Design review of the part built by this model. Coordinates are the model's own, in mm. A direction names the side the tool comes from. Coordinates: 2 decimals unless noted, no trailing zeros. Order: outer loops, then holes, each group sorted by start corner. A loop starts at its lowest first (then second) coordinate and runs counter-clockwise, first axis right, second up. Notation, with made-up numbers: M 82.25,-19.75 L 113.25,-19.75 A24 ccw 113.25,-8.75 Z; hole C 62.25,-13 d4. An arc over 180 degrees is marked long. Use CSV: the item, a comma, the result in double quotes.
```python
from build123d import *

# Parameters (mm, degrees)
ESQUISSE1_W             = 197
ESQUISSE1_H             = 55
BOSS_EXTRU_1_DEPTH      = 4
ESQUISSE3_R             = 1.5
ENL_V_MAT_EXTRU_2_DEPTH = 4
CHANFREIN1_SIZE         = 2
ESQUISSE4_W             = 160.5
ESQUISSE4_H             = 41.5
ENL_V_MAT_EXTRU_3_DEPTH = 10
ESQUISSE5_W             = 2
ESQUISSE5_H             = 41.395615901
ESQUISSE5_H_2           = 41.375
BOSS_EXTRU_2_DEPTH      = 20
ESQUISSE6_W             = 20
ESQUISSE6_H             = 2.5
BOSS_EXTRU_3_DEPTH      = 3
ESQUISSE7_W             = 20
ESQUISSE7_H             = 2.5
BOSS_EXTRU_4_DEPTH      = 3
CHANFREIN3_SIZE         = 4
CHANFREIN3_SIZE_2       = 10.989909678
ESQUISSE8_R             = 1.375
ENL_V_MAT_EXTRU_4_DEPTH = 900
CHANFREIN4_SIZE         = 1
ESQUISSE9_W             = 164.5
ESQUISSE9_H             = 3
BOSS_EXTRU_5_DEPTH      = 5


with BuildPart() as part:
    # Esquisse1 → Boss.-Extru.1 (new body)
    with BuildSketch(Plane.XY):
        with Locations((98.5, 27.5)):
            Rectangle(ESQUISSE1_W, ESQUISSE1_H)
    extrude(amount=BOSS_EXTRU_1_DEPTH)

    # Esquisse3 → Enlèv. mat.-Extru.2 (cut)
    with BuildSketch(Plane.XY.offset(4)):
        with Locations((4.25, 50.75)):
            Circle(ESQUISSE3_R)
        with Locations((4.25, 4.25)):
            Circle(ESQUISSE3_R)
        with Locations((192.75, 4.25)):
            Circle(ESQUISSE3_R)
        with Locations((192.75, 50.75)):
            Circle(ESQUISSE3_R)
    extrude(amount=-ENL_V_MAT_EXTRU_2_DEPTH, mode=Mode.SUBTRACT)

    # Chanfrein1
    chanfrein1_edges = [part.edges().sort_by_distance(p)[0] for p in [
        (2.75, 50.75, 4),
        (2.75, 4.25, 4),
        (191.25, 4.25, 4),
        (191.25, 50.75, 4),
    ]]
    chamfer(chanfrein1_edges, length=CHANFREIN1_SIZE)

    # Esquisse4 → Enlèv. mat.-Extru.3 (cut)
    with BuildSketch(Plane.XY.offset(4)):
        with Locations((98.5, 27.5)):
            Rectangle(ESQUISSE4_W, ESQUISSE4_H)
    extrude(amount=-ENL_V_MAT_EXTRU_3_DEPTH, mode=Mode.SUBTRACT)

    # Esquisse5 → Boss.-Extru.2 (add)
    with BuildSketch(Plane(origin=(0, 0, 0), x_dir=(-1, 0, 0), z_dir=(0, 0, -1))):
        with Locations((-17.25, 27.447807951)):
            Rectangle(ESQUISSE5_W, ESQUISSE5_H)
        with Locations((-179.75, 27.5625)):
            Rectangle(ESQUISSE5_W, ESQUISSE5_H_2)
    extrude(amount=BOSS_EXTRU_2_DEPTH)

    # Esquisse6 → Boss.-Extru.3 (add)
    with BuildSketch(Plane.ZY.offset(-178.75)):
        with Locations((-10, 18.375)):
            Rectangle(ESQUISSE6_W, ESQUISSE6_H)
        with Locations((-10, 36.75)):
            Rectangle(ESQUISSE6_W, ESQUISSE6_H)
    extrude(amount=BOSS_EXTRU_3_DEPTH)

    # Esquisse7 → Boss.-Extru.4 (add)
    with BuildSketch(Plane(origin=(18.25, 0, 0), x_dir=(0, 0, -1), z_dir=(1, 0, 0))):
        with Locations((10, 18.25)):
            Rectangle(ESQUISSE7_W, ESQUISSE7_H)
        with Locations((10, 36.645615901)):
            Rectangle(ESQUISSE7_W, ESQUISSE7_H)
    extrude(amount=BOSS_EXTRU_4_DEPTH)

    # Chanfrein3
    # the kernel refuses this chamfer: 10.989909678, 4 mm, written as the material it takes off along each edge
    with BuildSketch(Plane(origin=(21.25, 48.009965797, 0), x_dir=(-0.9950833631817486, 0, 0.0990409022520506), z_dir=(0, -1, 0))) as chanfrein3_piece_1_section:
        Polygon((CHANFREIN3_SIZE * 0.995083363182, CHANFREIN3_SIZE * 0.0990409022521), (-CHANFREIN3_SIZE_2 * 0.0990409022504, CHANFREIN3_SIZE_2 * 0.995083363165), (0, 0), align=None)
    chanfrein3_piece_1 = extrude(amount=59.519931595, mode=Mode.PRIVATE)
    chanfrein3_piece_1 = split(chanfrein3_piece_1, bisect_by=Plane(origin=(18.25, 18.25, -4.010147901), z_dir=(1, 0, 0)), keep=Keep.TOP, mode=Mode.PRIVATE)
    add(chanfrein3_piece_1, mode=Mode.SUBTRACT)
    with BuildSketch(Plane(origin=(21.25, 6.885650104, 0), x_dir=(-0.9950833631817486, 0, 0.0990409022520506), z_dir=(0, 1, 0))) as chanfrein3_piece_2_section:
        Polygon((CHANFREIN3_SIZE * 0.995083363182, -CHANFREIN3_SIZE * 0.0990409022521), (-CHANFREIN3_SIZE_2 * 0.0990409022504, -CHANFREIN3_SIZE_2 * 0.995083363165), (0, 0), align=None)
    chanfrein3_piece_2 = extrude(amount=59.519931595, mode=Mode.PRIVATE)
    chanfrein3_piece_2 = split(chanfrein3_piece_2, bisect_by=Plane(origin=(18.25, 36.645615901, -4.010147901), z_dir=(1, 0, 0)), keep=Keep.TOP, mode=Mode.PRIVATE)
    add(chanfrein3_piece_2, mode=Mode.SUBTRACT)
    with BuildSketch(Plane(origin=(175.75, 66.509965797, 0), x_dir=(0.9950833631817486, 0, 0.09904090225205044), z_dir=(0, -1, 0))) as chanfrein3_piece_3_section:
        Polygon((CHANFREIN3_SIZE * 0.995083363182, -CHANFREIN3_SIZE * 0.0990409022521), (-CHANFREIN3_SIZE_2 * 0.0990409022504, -CHANFREIN3_SIZE_2 * 0.995083363165), (0, 0), align=None)
    chanfrein3_piece_3 = extrude(amount=59.519931595, mode=Mode.PRIVATE)
    chanfrein3_piece_3 = split(chanfrein3_piece_3, bisect_by=Plane(origin=(178.75, 36.75, -4.010147901), z_dir=(-1, 0, 0)), keep=Keep.TOP, mode=Mode.PRIVATE)
    add(chanfrein3_piece_3, mode=Mode.SUBTRACT)
    with BuildSketch(Plane(origin=(175.75, 48.134965797, 0), x_dir=(0.9950833631817486, 0, 0.09904090225205044), z_dir=(0, -1, 0))) as chanfrein3_piece_4_section:
        Polygon((CHANFREIN3_SIZE * 0.995083363182, -CHANFREIN3_SIZE * 0.0990409022521), (-CHANFREIN3_SIZE_2 * 0.0990409022504, -CHANFREIN3_SIZE_2 * 0.995083363165), (0, 0), align=None)
    chanfrein3_piece_4 = extrude(amount=59.519931595, mode=Mode.PRIVATE)
    chanfrein3_piece_4 = split(chanfrein3_piece_4, bisect_by=Plane(origin=(178.75, 18.375, -4.010147901), z_dir=(-1, 0, 0)), keep=Keep.TOP, mode=Mode.PRIVATE)
    add(chanfrein3_piece_4, mode=Mode.SUBTRACT)

    # Esquisse8 → Enlèv. mat.-Extru.4 (cut)
    with BuildSketch(Plane(origin=(180.75, 0, 0), x_dir=(0, 0, -1), z_dir=(1, 0, 0))):
        with Locations((5, 27.62)):
            Circle(ESQUISSE8_R)
    extrude(amount=-ENL_V_MAT_EXTRU_4_DEPTH, mode=Mode.SUBTRACT)

    # Chanfrein4
    chanfrein4_edges = [part.edges().sort_by_distance(p)[0] for p in [
        (16.25, 27.62, -3.625),
        (180.75, 27.62, -3.625),
    ]]
    chamfer(chanfrein4_edges, length=CHANFREIN4_SIZE)

    # Esquisse9 → Boss.-Extru.5 (add)
    with BuildSketch(Plane(origin=(0, 0, 0), x_dir=(-1, 0, 0), z_dir=(0, 0, -1))):
        with Locations((-98.5, 52)):
            Rectangle(ESQUISSE9_W, ESQUISSE9_H)
        with Locations((-98.5, 3)):
            Rectangle(ESQUISSE9_W, ESQUISSE9_H)
    extrude(amount=BOSS_EXTRU_5_DEPTH)


solid = part.part
```
(1) Add section B-B on z = -14.25. State the section outline as (x, y) points (3 decimals).
The answers:
outline,"M 16.25,6.75 L 18.25,6.75 L 18.25,17 L 21.25,17 L 21.25,19.5 L 18.25,19.5 L 18.25,35.396 L 21.25,35.396 L 21.25,37.896 L 18.25,37.896 L 18.25,48.146 L 16.25,48.146 Z; M 175.75,17.125 L 178.75,17.125 L 178.75,6.875 L 180.75,6.875 L 180.75,48.25 L 178.75,48.25 L 178.75,38 L 175.75,38 L 175.75,35.5 L 178.75,35.5 L 178.75,19.625 L 175.75,19.625 Z"
(2) Wall thickness on probe 1 along Y at (x, z) = (4.25, 0.7); probe 2 along X at (y, z) = (7, -1.75); probe 3 along Y at (x, z) = (75.5, -4): over which ranges is each line inside the solid? List them lowest first.
The answers:
probe 1,"y = 0 to 2.75, 5.75 to 49.25, 52.25 to 55"
probe 2,"x = 16.25 to 18.25, 178.75 to 180.75"
probe 3,"y = 1.5 to 4.5, 50.5 to 53.5"
(3) For faces 1 (the face through (100, 1.5, -2)), 2 (the face through (97, 6.75, 2)), 3 (the face through (16.25, 27, -10)), 4 (the face through (98, 5, 0)), list the 3-axis set-ups (+Z, -Z, +X, -X, +Y, -Y) from which the entire face can be reached by the end or side of a thin tool; tool diameter is ignored.
The answers:
face 1,"-Z, +X, -X, -Y"
face 2,"+Z, -Z"
face 3,"-Z, -X, +Y, -Y"
face 4,"-Z"
(4) Add section A-A on y = 13. State the section outline as (x, z) points.
The answers:
outline,"M 0,0 L 16.25,0 L 16.25,-20 L 18.25,-20 L 18.25,4 L 0,4 Z; M 178.75,-20 L 180.75,-20 L 180.75,0 L 197,0 L 197,4 L 178.75,4 Z"
(5) Clearance check with flat-ended pins moving along their axes: P1, Ø6, axis at x = 150.5, y = 48, coming from the -Z side; P2, Ø3.5, axis at x = 177.5, z = -8, coming from the -Y side (3 decimals); P3, Ø2.5, axis at y = 27.62, z = -5, coming from the -X side; P4, Ø10, axis at y = 25, z = -6.5, coming from the +X side. State where each tip first meets the part, or that it passes through.
The answers:
P1,"stops at z = -5"
P2,"stops at y = 6.875"
P3,"passes through"
P4,"stops at x = 180.75"
(6) Add section C-C on x = 72. State the section outline as (y, z) points.
The answers:
outline,"M 0,0 L 1.5,0 L 1.5,-5 L 4.5,-5 L 4.5,0 L 6.75,0 L 6.75,4 L 0,4 Z; M 48.25,0 L 50.5,0 L 50.5,-5 L 53.5,-5 L 53.5,0 L 55,0 L 55,4 L 48.25,4 Z"
